Input: part model. Units: mm. Frame: model coordinates. A direction names the side the tool comes from. Coordinates: 2 decimals unless noted, no trailing zeros. Loops run counter-clockwise (first coordinate to the right, second up) from the corner with the lowest first, then second, coordinate; pieces in that order, holes last. Notation, with made-up numbers: (84, 62.25) - (134, 62.25) arc R21 ccw to (134, 100.25) - close; hole circle Ø9 at (6, 76.5). An arc over 180 degrees is marked (long way). Use a Markdown table: item, result. Add a question column.
1. Section query B-B on y = 38. Return the cut outline in (x, z), then the cut area to 3 significant figures.
2. Ray query, L1, parallel to X at y = -2.2, z = -10; L2, parallel to Z at x = -37, y = 39.5; L3, parallel to Z at x = -16, y = 35. Return the intervals inside material, ascending. Write a range as [from, to].
3. Section query C-C on x = -33.5. Return the cut outline in (y, z).
4. Section query A-A on y = 21. Return the cut outline in (x, z), then the cut area to 3 significant figures.
5. Draft query along X for faces 5 (the face through (29.131, 18.846, 32.77)), 6 (the face through (-43.635, 28, 19)), 7 (the face through (14, -2.764, -11)), 8 (the face through (13.079, 5.405, 32.605)). Return one class per face: released by +X, released by -X, zero draft, split by the parting line, or undercut.
6. Contact query for flat-ended pins moving along their axis: P1, Ø13.5, axis at y = 54.5, z = 9, coming from the -X side; P2, Ø4.5, axis at x = -2.74, z = -10, coming from the +Y side; P3, Ø25, axis at x = -24.5, z = 8, coming from the +Y side. Output: stop coordinate, or through.
7. Access query for faces 1 (the face through (-31.948, 54, 14)), 2 (the face through (30.044, -1.835, -9.239)), 3 (the face through (40, 13, 0)), 4 (the face through (36.04, 74.34, -44.04)). Directions: +Z, -Z, +X, -X, +Y, -Y. A direction counts if a zero-diameter tool reaches every point of the face in a straight line with its end or side. Return the directions, or none.
```python
from build123d import *

# Parameters (mm, degrees)
EXTRUDE_9_DEPTH          = 27.7
EXTRUDE_START            = 15
EXTRUDE_10_DEPTH         = 15
SKETCH_9_W               = 120
SKETCH_9_H               = 10
EXTRUDE_11_DEPTH         = 27.7
SKETCH_10_R              = 29.5
EXTRUDE_14_DEPTH         = 27.7
EXTRUDE_15_DEPTH         = 10
SKETCH_12_R              = 32
CUT_EXTRUDE_1_DEPTH      = 10
PATTERN_CIRCULAR_1_COUNT = 8
PATTERN_CIRCULAR_2_COUNT = 6


with BuildPart() as part:
    # 草图1 → 凸台-拉伸9 (new body)
    with BuildSketch(Plane.XY):
        with BuildLine():
            Line((-45.634664851, -2.764128119), (74.365335149, -2.764128119))
            Line((74.365335149, -2.764128119), (74.365335149, 7.235871881))
            Line((74.365335149, 7.235871881), (72.365335149, 7.235871881))
            Line((72.365335149, 7.235871881), (72.365335149, 47.235871881))
            ThreePointArc((72.365335149, 47.235871881), (14.365335149, 105.235871881), (-43.634664851, 47.235871881))
            Line((-43.634664851, 47.235871881), (-43.634664851, 7.235871881))
            Line((-43.634664851, 7.235871881), (-45.634664851, 7.235871881))
            Line((-45.634664851, 7.235871881), (-45.634664851, -2.764128119))
        make_face()
        with BuildLine():
            Line((-31.9477266, 40.650970024), (-31.9477266, 68.146424194))
            ThreePointArc((-31.9477266, 68.146424194), (14.3022734, 102.648697109), (60.5522734, 68.146424194))
            Line((60.5522734, 68.146424194), (60.5522734, 40.650970024))
            ThreePointArc((60.5522734, 40.650970024), (14.3022734, 6.148697109), (-31.9477266, 40.650970024))
        make_face(mode=Mode.SUBTRACT)
    extrude(amount=EXTRUDE_9_DEPTH)

    # 草图8 → 凸台-拉伸10 (add)
    with BuildSketch(Plane(origin=(0, 0, 0), x_dir=(-1, 0, 0), z_dir=(0, 0, -1)).offset(EXTRUDE_START)):
        with BuildLine():
            Line((-74.365335149, -2.764128119), (45.634664851, -2.764128119))
            Line((45.634664851, -2.764128119), (45.634664851, 7.235871881))
            Line((45.634664851, 7.235871881), (-4.117460368, 7.235871881))
            ThreePointArc((-4.117460368, 7.235871881), (-14.3022734, 6.148697109), (-24.487086433, 7.235871881))
            Line((-24.487086433, 7.235871881), (-74.365335149, 7.235871881))
            Line((-74.365335149, 7.235871881), (-74.365335149, -2.764128119))
        make_face()
    extrude_10 = extrude(amount=-EXTRUDE_10_DEPTH)

    # 镜向4: 凸台-拉伸10 across plane
    add(extrude_10.mirror(Plane(origin=(0, 0, -15), x_dir=(1, 0, 0), z_dir=(0, 0, -1))))

    # 草图9 → 凸台-拉伸11 (add)
    with BuildSketch(Plane(origin=(0, 0, -30), x_dir=(-1, 0, 0), z_dir=(0, 0, -1))):
        with Locations((-14.365335149, 2.235871881)):
            Rectangle(SKETCH_9_W, SKETCH_9_H)
    extrude(amount=EXTRUDE_11_DEPTH)

    # 草图10 → 凸台-拉伸14 (add)
    with BuildSketch(Plane(origin=(0, 0, -57.7), x_dir=(-1, 0, 0), z_dir=(0, 0, -1))):
        with BuildLine():
            Line((-72.365335149, 47.235871881), (-72.365335149, 7.235871881))
            Line((-72.365335149, 7.235871881), (43.634664851, 7.235871881))
            Line((43.634664851, 7.235871881), (43.634664851, 47.235871881))
            ThreePointArc((43.634664851, 47.235871881), (-14.365335149, 105.235871881), (-72.365335149, 47.235871881))
        make_face()
        with Locations((-14.3022734, 54.398697109)):
            Circle(SKETCH_10_R, mode=Mode.SUBTRACT)
    extrude(amount=-EXTRUDE_14_DEPTH)

    # 草图11 → 凸台-拉伸15 (add)
    with BuildSketch(Plane.XY.offset(27.7)):
        with BuildLine():
            Line((-45.634664851, 7.235871881), (-45.634664851, -2.764128119))
            Line((-45.634664851, -2.764128119), (74.365335149, -2.764128119))
            Line((74.365335149, -2.764128119), (74.365335149, 7.235871881))
            Line((74.365335149, 7.235871881), (72.365335149, 7.235871881))
            Line((72.365335149, 7.235871881), (72.365335149, 47.235871881))
            ThreePointArc((72.365335149, 47.235871881), (14.365335149, 105.235871881), (-43.634664851, 47.235871881))
            Line((-43.634664851, 47.235871881), (-43.634664851, 7.235871881))
            Line((-43.634664851, 7.235871881), (-45.634664851, 7.235871881))
        make_face()
    extrude(amount=EXTRUDE_15_DEPTH)

    # 草图12 → 切除-拉伸1 (cut)
    with BuildSketch(Plane.XY.offset(37.7)):
        with Locations((14.365335149, 47.235871881)):
            Circle(SKETCH_12_R)
    extrude(amount=-CUT_EXTRUDE_1_DEPTH, mode=Mode.SUBTRACT)

    # 草图22 → M3.5 螺纹孔5 (revolve, cut)
    with BuildSketch(Plane(origin=(14.365335149, 89.735871881, 37.7), x_dir=(0, -1, 0), z_dir=(1, 0, 0))):
        Polygon((0, 0), (0, 10.871247898), (1.45, 10), (1.45, 0.325), (1.775, 0), align=None)
    hole_wizard_m3_5_5 = revolve(axis=Axis((14.365335149, 89.735871881, 44.05), (0, 0, -1)), mode=Mode.SUBTRACT)

    # 阵列(圆周)1: M3.5 螺纹孔5 ×8 about axis
    pattern_circular_1_axis = Axis((14.365335149, 47.235871881, 0), (0, 0, 1))
    for i in range(1, PATTERN_CIRCULAR_1_COUNT):
        add(hole_wizard_m3_5_5.rotate(pattern_circular_1_axis, i * 360 / PATTERN_CIRCULAR_1_COUNT), mode=Mode.SUBTRACT)

    # 草图25 → M4 螺纹孔1 (revolve, cut)
    with BuildSketch(Plane(origin=(-2.738231277, -2.764128119, -10), x_dir=(0, 0, -1), z_dir=(1, 0, 0))):
        Polygon((0, 0), (0, 2.491420021), (1.65, 1.5), (1.65, 0.375), (2.025, 0), align=None)
    hole_wizard_m4_1 = revolve(axis=Axis((-2.738231277, -9.114128119, -10), (0, 1, 0)), mode=Mode.SUBTRACT)

    # 阵列(圆周)2: M4 螺纹孔1 ×6 about axis
    pattern_circular_2_axis = Axis((14.384603563, 0, -10), (0, 1, 0))
    for i in range(1, PATTERN_CIRCULAR_2_COUNT):
        add(hole_wizard_m4_1.rotate(pattern_circular_2_axis, i * 360 / PATTERN_CIRCULAR_2_COUNT), mode=Mode.SUBTRACT)


solid = part.part
```
Resolved:
| question | item | result |
|---|---|---|
| 1 | outline | (-43.63, -57.7) - (-10.22, -57.7) - (-10.22, -30) - (-43.63, -30) - close; (-43.63, 0) - (-31.08, 0) - (-31.08, 27.7) - (-16.27, 27.7) - (-16.27, 37.7) - (-43.63, 37.7) - close; (38.82, -57.7) - (72.37, -57.7) - (72.37, -30) - (38.82, -30) - close; (45, 27.7) - (59.68, 27.7) - (59.68, 0) - (72.37, 0) - (72.37, 37.7) - (45, 37.7) - close |
| 1 | area | 3,100 mm² |
| 2 | L1 | [-45.63, -4.39], [-1.09, 29.86], [33.16, 74.37] |
| 2 | L2 | [-57.7, -30], [0, 37.7] |
| 2 | L3 | [-57.7, -30], [27.7, 37.7] |
| 3 | outline | (-2.76, -57.7) - (79.99, -57.7) - (79.99, -30) - (7.24, -30) - (7.24, 0) - (79.99, 0) - (79.99, 37.7) - (-2.76, 37.7) - close |
| 4 | outline | (-43.63, -57.7) - (72.37, -57.7) - (72.37, -30) - (-43.63, -30) - close; (-43.63, 0) - (-20.52, 0) - (-20.52, 27.7) - (-3.96, 27.7) - (-3.96, 37.7) - (-43.63, 37.7) - close; (32.69, 27.7) - (49.12, 27.7) - (49.12, 0) - (72.37, 0) - (72.37, 37.7) - (32.69, 37.7) - close |
| 4 | area | 5,290 mm² |
| 5 | face 5 | undercut |
| 5 | face 6 | released by -X |
| 5 | face 7 | zero draft |
| 5 | face 8 | undercut |
| 6 | P1 | x = -43.63 |
| 6 | P2 | y = 7.24 |
| 6 | P3 | y = 98.9 |
| 7 | face 1 | none |
| 7 | face 2 | -Y |
| 7 | face 3 | +X, -X, +Y |
| 7 | face 4 | -Z |
